For this review, use the dimensioned drawing (mm, ordinates from the lowest corner) and the shaded views. A direction names the side the tool comes from. Coordinates: 2 decimals unless noted, no trailing zeros. Order: outer loops, then holes, each group sorted by start corner. A loop starts at its lowest first (then second) coordinate and runs counter-clockwise, first axis right, second up. Notation, with made-up numbers: (-17, -24.75) -> (20, -24.75) arc R22 cw to (20, 4.25) -> close; hole circle Ø1 at (80.25, -36.5). An arc over 180 degrees is marked (long way). Return JSON: item names as keys, results as strings. Group by question number.
Item 1: Take a section at A-A (y = 39.5). Write out the cut boundary in (x, z), then the cut area to 3 significant figures.
Item 2: Take a section at D-D (z = 40). Write out the cut boundary in (x, y), then the cut area to 3 significant figures.
Item 3: Insertion check: pin 1 (2 mm diameter, centred on x = 17.5, z = 6.5, fed in from -Y); pin 2 (6 mm diameter, centred on x = 12, z = 38.5, fed in from +Y). Each pin has a flat end and moves straight along its axis. Give the tip position at first contact, or say it passes through.
Item 4: Draft analysis for pull direction X (two halves, no side actions). For the marked faces 1, 2 and 3, state which applies: +X half, -X half, draft (parallel to the pull), parting line (faces both ways), or undercut.
Item 5: Take a section at C-C (x = 17.5). Write out the cut boundary in (y, z).
Item 6: Machinability: for the marked faces 4 and 5, which of the approach directions +Z, -Z, +X, -X, +Y, -Y give a long, thin tool a straight path to every point of the face, cutting with its end or side? Answer none if there is none.
Item 7: Take a section at B-B (z = 25). Write out the cut boundary in (x, y).
Item 8: For line 1 along X through (y, z) = (19, 26.5); line 2 along Y through (x, z) = (17.5, 35); line 3 along Y through (x, z) = (18, 32), list the stretches that pass through material, from the lowest coordinate up.
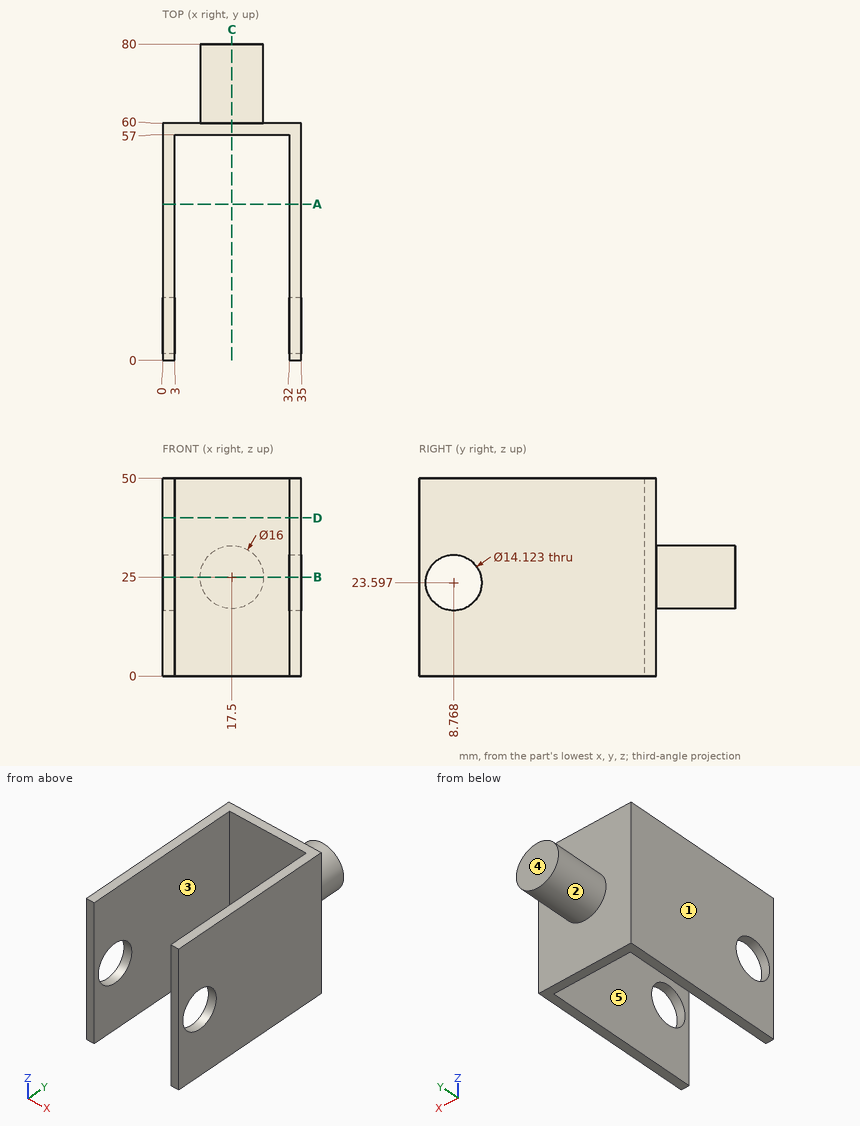
Findings below:
{
 "1": {"outline": "(0, 0) -> (3, 0) -> (3, 50) -> (0, 50) -> close; (32, 0) -> (35, 0) -> (35, 50) -> (32, 50) -> close", "area": "300 mm2"},
 "2": {"outline": "(0, 0) -> (3, 0) -> (3, 57) -> (32, 57) -> (32, 0) -> (35, 0) -> (35, 60) -> (0, 60) -> close", "area": "447 mm2"},
 "3": {"pin 1": "stops at y = 57", "pin 2": "stops at y = 60"},
 "4": {"face 1": "-X half", "face 2": "parting line", "face 3": "undercut"},
 "5": {"outline": "(57, 0) -> (60, 0) -> (60, 17) -> (80, 17) -> (80, 33) -> (60, 33) -> (60, 50) -> (57, 50) -> close"},
 "6": {"face 4": "+Z, -Z, +X, -X, +Y", "face 5": "+Z, -Z, -Y"},
 "7": {"outline": "(0, 0) -> (3, 0) -> (3, 1.85) -> (0, 1.85) -> close; (0, 15.69) -> (3, 15.69) -> (3, 57) -> (32, 57) -> (32, 15.69) -> (35, 15.69) -> (35, 60) -> (25.5, 60) -> (25.5, 80) -> (9.5, 80) -> (9.5, 60) -> (0, 60) -> close; (32, 0) -> (35, 0) -> (35, 1.85) -> (32, 1.85) -> close"},
 "8": {"line 1": "x = 0 to 3, 32 to 35", "line 2": "y = 57 to 60", "line 3": "y = 57 to 80"}
}
